from build123d import *

# Parameters (mm, degrees)
SKETCH1_R           = 5.75
BOSS_EXTRUDE1_DEPTH = 4
SKETCH6_R           = 9.5
CUT_EXTRUDE1_DEPTH  = 5


with BuildPart() as part:
    # Sketch1 → Boss-Extrude1 (new body)
    with BuildSketch(Plane(origin=(0, 0, 0), x_dir=(1, 0, 0), z_dir=(0, 1, 0))):
        with BuildLine():
            Line((14.722227154, 13.97), (29.21, 13.97))
            ThreePointArc((29.21, 13.97), (33.700128061, 12.110128061), (35.56, 7.62))
            Line((35.56, 7.62), (35.56, -7.62))
            ThreePointArc((35.56, -7.62), (33.700128061, -12.110128061), (29.21, -13.97))
            Line((29.21, -13.97), (19.176579466, -13.97))
            ThreePointArc((19.176579466, -13.97), (16.831686562, -14.418815604), (14.818265951, -15.701818182))
            ThreePointArc((14.818265951, -15.701818182), (0, -21.59), (-14.818265951, -15.701818182))
            ThreePointArc((-14.818265951, -15.701818182), (-16.831686562, -14.418815604), (-19.176579466, -13.97))
            Line((-19.176579466, -13.97), (-29.21, -13.97))
            ThreePointArc((-29.21, -13.97), (-33.700128061, -12.110128061), (-35.56, -7.62))
            Line((-35.56, -7.62), (-35.56, 7.62))
            ThreePointArc((-35.56, 7.62), (-33.700128061, 12.110128061), (-29.21, 13.97))
            Line((-29.21, 13.97), (-14.722227154, 13.97))
            ThreePointArc((-14.722227154, 13.97), (-13.078726217, 13.753628997), (-11.547227154, 13.119261314))
            Line((-11.547227154, 13.119261314), (-8.995011096, 11.645738686))
            ThreePointArc((-8.995011096, 11.645738686), (-7.463512032, 11.011371003), (-5.820011096, 10.795))
            Line((-5.820011096, 10.795), (5.820011096, 10.795))
            ThreePointArc((5.820011096, 10.795), (7.463512032, 11.011371003), (8.995011096, 11.645738686))
            Line((8.995011096, 11.645738686), (11.547227154, 13.119261314))
            ThreePointArc((11.547227154, 13.119261314), (13.078726217, 13.753628997), (14.722227154, 13.97))
        make_face()
        Circle(SKETCH1_R, mode=Mode.SUBTRACT)
        with BuildLine():
            Line((-23.495, -2.667), (-29.21, -2.667))
            ThreePointArc((-29.21, -2.667), (-31.877, 0), (-29.21, 2.667))
            Line((-29.21, 2.667), (-23.495, 2.667))
            ThreePointArc((-23.495, 2.667), (-20.828, 0), (-23.495, -2.667))
        make_face(mode=Mode.SUBTRACT)
        with BuildLine():
            Line((23.495, 2.667), (29.21, 2.667))
            ThreePointArc((29.21, 2.667), (31.877, 0), (29.21, -2.667))
            Line((29.21, -2.667), (23.495, -2.667))
            ThreePointArc((23.495, -2.667), (20.828, 0), (23.495, 2.667))
        make_face(mode=Mode.SUBTRACT)
        with BuildLine():
            Line((-15.289419162, 6.517949192), (-13.089714637, 5.247949192))
            ThreePointArc((-13.089714637, 5.247949192), (-10.357663829, 5.98), (-11.089714637, 8.712050808))
            Line((-11.089714637, 8.712050808), (-13.289419162, 9.982050808))
            ThreePointArc((-13.289419162, 9.982050808), (-16.02146997, 9.25), (-15.289419162, 6.517949192))
        make_face(mode=Mode.SUBTRACT)
        with BuildLine():
            Line((13.289419162, 9.982050808), (11.089714637, 8.712050808))
            ThreePointArc((11.089714637, 8.712050808), (10.357663829, 5.98), (13.089714637, 5.247949192))
            Line((13.089714637, 5.247949192), (15.289419162, 6.517949192))
            ThreePointArc((15.289419162, 6.517949192), (16.02146997, 9.25), (13.289419162, 9.982050808))
        make_face(mode=Mode.SUBTRACT)
        with BuildLine():
            Line((2, -16.5), (2, -13.96))
            ThreePointArc((2, -13.96), (0, -11.96), (-2, -13.96))
            Line((-2, -13.96), (-2, -16.5))
            ThreePointArc((-2, -16.5), (0, -18.5), (2, -16.5))
        make_face(mode=Mode.SUBTRACT)
    extrude(amount=BOSS_EXTRUDE1_DEPTH)

    # Sketch6 → Cut-Extrude1 (cut, through all)
    with BuildSketch(Plane(origin=(0, 4, 0), x_dir=(1, 0, 0), z_dir=(0, 1, 0))):
        Circle(SKETCH6_R)
    extrude(amount=-CUT_EXTRUDE1_DEPTH, mode=Mode.SUBTRACT)


solid = part.part
Model file for the job. Use its own axes, mm. A direction names the side the tool comes from. Round coordinates to 2 decimals unless told otherwise and drop trailing zeros. Order: outer loops, then holes, each group sorted by start corner. A loop starts at its lowest first (then second) coordinate and runs counter-clockwise, first axis right, second up.
(1) Pin check, flat tips, straight feed: pin 1 (2 mm diameter, centred on y = 1.5, z = 13.5, fed in from +X); pin 2 (1.2 mm diameter, centred on x = -26, y = 3, fed in from +Z); pin 3 (2 mm diameter, centred on x = -1.5, y = 2, fed in from -Z) (3 decimals). Stop position of each tip, or through.
(2) Drill centre lines: line 1 (X direction, y = 0.9, z = 0); line 2 (Z direction, x = 0, y = 1.3) (3 decimals); line 3 (Z direction, x = 24, y = 2.95). Where is each one in solid material? Low to high.
(3) Band-saw the part on A-A (x = 27). List the corners of the cut face in (y, z).
(4) Pull direction Z, two halves, no side cores. Call faces 1 (the face through (0.04, 1.97, 11.96)), 2 (the face through (10.3, 2, -12.4)), 3 (the face through (26, 2, -2.667)), 4 (the face through (33.75, 1.97, 12.06)): released by +Z, released by -Z, zero draft, split by the parting line, or undercut.
(5) Band-saw the part on D-D (y = 1.8). Give the number of separate pieces and of enclosed holes in the cut face, then the cut area to 3 significant figures.
(6) Band-saw the part on C-C (x = 0). List the corners of the cut face in (y, z) (3 decimals).
(7) 3-axis set-ups, long thin cutter, end or side, ignore diameter. For faces 5 (the face through (-33.75, 1.97, -12.06)), 6 (the face through (-13.1, 1.97, -13.76)), 7 (the face through (0, 2, 18.5)): which of +Z, -Z, +X, -X, +Y, -Y reach the whole face in a straight line?
(8) Band-saw the part on B-B (z = 2). List the corners of the cut face in (x, y), then the cut area to 3 significant figures.
Verdict:
1. pin 1: stops at x = 33.27
1. pin 2: stops at z = 13.97
1. pin 3: stops at z = -10.795
2. line 1: x = -35.56 to -31.88, -20.83 to -9.5, 9.5 to 20.83, 31.88 to 35.56
2. line 2: z = -10.795 to -9.5, 9.5 to 11.96, 18.5 to 21.59
2. line 3: z = -13.97 to -2.67, 2.67 to 13.97
3. outline: (0, -13.97) - (4, -13.97) - (4, -2.67) - (0, -2.67) - close; (0, 2.67) - (4, 2.67) - (4, 13.97) - (0, 13.97) - close
4. face 1: undercut
4. face 2: released by -Z
4. face 3: undercut
4. face 4: released by +Z
5. separate pieces: 1
5. enclosed holes: 6
5. area: 1,610 mm2
6. outline: (0, -10.795) - (4, -10.795) - (4, -9.5) - (0, -9.5) - close; (0, 9.5) - (4, 9.5) - (4, 11.96) - (0, 11.96) - close; (0, 18.5) - (4, 18.5) - (4, 21.59) - (0, 21.59) - close
7. face 5: -Z, -X, +Y, -Y
7. face 6: -Z, +Y, -Y
7. face 7: +Y, -Y
8. outline: (-35.56, 0) - (-30.97, 0) - (-30.97, 4) - (-35.56, 4) - close; (-21.73, 0) - (-9.29, 0) - (-9.29, 4) - (-21.73, 4) - close; (9.29, 0) - (21.73, 0) - (21.73, 4) - (9.29, 4) - close; (30.97, 0) - (35.56, 0) - (35.56, 4) - (30.97, 4) - close
8. area: 136 mm2
